```python
from build123d import *

# Parameters (mm, degrees)
SKETCH1_R               = 17.5
BOSS_EXTRUDE1_DEPTH     = 30
SKETCH5_R               = 10.95
CUT_EXTRUDE2_DEPTH      = 39.890873
SWEEP2_PITCH            = 10
SKETCH8_R               = 17.5
CUT_EXTRUDE3_DEPTH      = 41.699
SKETCH9_R               = 17.5
CUT_EXTRUDE4_DEPTH      = 39.890874
SKETCH10_W              = 40
SKETCH10_H              = 19.977262
BOSS_EXTRUDE2_DEPTH     = 40
SKETCH11_W              = 40
SKETCH11_H              = 19.977262
BOSS_EXTRUDE3_DEPTH     = 10
BOSS_EXTRUDE4_DEPTH     = 30
SKETCH14_R              = 1.905
CUT_EXTRUDE5_DEPTH      = 71.869594
SKETCH15_R              = 3.9243
CUT_EXTRUDE7_DEPTH      = 59.798031
SKETCH16_W              = 50
SKETCH16_H              = 19.977262
BOSS_EXTRUDE5_DEPTH     = 22
CUT_EXTRUDE8_DEPTH      = 12
BOSS_EXTRUDE6_DEPTH     = 19.977262
BOSS_EXTRUDE7_DEPTH     = 22
FILLET1_R               = 2
SKETCH21_W              = 7
SKETCH21_H              = 16
BOSS_EXTRUDE8_DEPTH     = 2
CUT_EXTRUDE9_DEPTH      = 76.769387
CUT_EXTRUDE9_DEPTH_BACK = 76.769387
SKETCH22_W              = 37.5
SKETCH22_H              = 30
SKETCH24_W              = 37.5
SKETCH24_H              = 30
BOSS_EXTRUDE9_DEPTH     = 12


with BuildPart() as part:
    # Sketch1 → Boss-Extrude1 (new body)
    with BuildSketch(Plane.XY):
        Circle(SKETCH1_R)
    extrude(amount=BOSS_EXTRUDE1_DEPTH)

    # Sketch5 → Cut-Extrude2 (cut, through all)
    with BuildSketch(Plane(origin=(0, 0, 0), x_dir=(-1, 0, 0), z_dir=(0, 0, -1))):
        Circle(SKETCH5_R)
    extrude(amount=-CUT_EXTRUDE2_DEPTH, mode=Mode.SUBTRACT)

    # Sweep2: arcs per turn and ends read off the stored shape
    # Sweep2: the profile of Sketch7 profile screwed along a right-hand helix through 3.75 turns, 16 arcs to a turn; built about Z, then put on its axis
    sweep2_z = Axis((0, 0, 0), (0, 0, 1))
    sweep2_corners = [(0, 7.7, 2.933013), (0, 10.9503, 4.809574), (0, 10.9503, 0.190426), (0, 7.7, 2.066987), (0, 7.45, 2.5)]
    with BuildLine(mode=Mode.PRIVATE) as sweep2_profile:
        Line(sweep2_corners[0], sweep2_corners[1])
        Line(sweep2_corners[1], sweep2_corners[2])
        Line(sweep2_corners[2], sweep2_corners[3])
        ThreePointArc((0, 7.7, 2.066987), (0, 7.516988, 2.25), (0, 7.45, 2.5))
        ThreePointArc((0, 7.45, 2.5), (0, 7.516988, 2.75), (0, 7.7, 2.933013))
    sweep2_cap = Face(sweep2_profile.wire())
    sweep2_arcs = [((0, 7.7, 2.066987), (0, 7.45, 2.211325), (0, 7.45, 2.5), (1, 0.8660254037844395, 1)), ((0, 7.45, 2.5), (0, 7.45, 2.788675), (0, 7.7, 2.933013), (1, 0.8660254037844395, 1))]  # start, shoulder, end, weights
    sweep2_turn_angles = [0, 11.25, 22.5, 33.75, 45, 56.25, 67.5, 78.75, 90, 101.25, 112.5, 123.75, 135, 146.25, 157.5, 168.75, 180, 191.25, 202.5, 213.75, 225, 236.25, 247.5, 258.75, 270, 281.25, 292.5, 303.75, 315, 326.25, 337.5, 348.75, 360]
    sweep2_turn_weights = [1, 0.9807852804032304, 1, 0.9807852804032304, 1, 0.9807852804032304, 1, 0.9807852804032304, 1, 0.9807852804032304, 1, 0.9807852804032304, 1, 0.9807852804032304, 1, 0.9807852804032304, 1, 0.9807852804032304, 1, 0.9807852804032304, 1, 0.9807852804032304, 1, 0.9807852804032304, 1, 0.9807852804032304, 1, 0.9807852804032304, 1, 0.9807852804032304, 1, 0.9807852804032304, 1]
    sweep2_turn_rails = [Edge.make_bspline([Vector(p[0], p[1], 0).rotate(sweep2_z, sweep2_turn_angles[k]) / sweep2_turn_weights[k] + Vector(0, 0, p[2] + SWEEP2_PITCH * sweep2_turn_angles[k] / 360) for k in range(33)], [0, 0, 0, 1, 1, 2, 2, 3, 3, 4, 4, 5, 5, 6, 6, 7, 7, 8, 8, 9, 9, 10, 10, 11, 11, 12, 12, 13, 13, 14, 14, 15, 15, 16, 16, 16], 2, sweep2_turn_weights) for p in sweep2_corners]
    sweep2_turn_sides = [*[Face.make_surface_from_curves(sweep2_turn_rails[p[0]], sweep2_turn_rails[p[1]]) for p in [(0, 1), (1, 2), (2, 3)]], *[Face.make_bezier_surface([[Vector(p[j][0], p[j][1], 0).rotate(sweep2_z, sweep2_turn_angles[2 * i + k]) / sweep2_turn_weights[2 * i + k] + Vector(0, 0, p[j][2] + SWEEP2_PITCH * sweep2_turn_angles[2 * i + k] / 360) for k in range(3)] for j in range(3)], [[p[3][j] * sweep2_turn_weights[2 * i + k] for k in range(3)] for j in range(3)]) for p in sweep2_arcs for i in range(16)]]
    sweep2_last_angles = [1080, 1091.25, 1102.5, 1113.75, 1125, 1136.25, 1147.5, 1158.75, 1170, 1181.25, 1192.5, 1203.75, 1215, 1226.25, 1237.5, 1248.75, 1260, 1271.25, 1282.5, 1293.75, 1305, 1316.25, 1327.5, 1338.75, 1350]
    sweep2_last_weights = [1, 0.9807852804032304, 1, 0.9807852804032304, 1, 0.9807852804032304, 1, 0.9807852804032304, 1, 0.9807852804032304, 1, 0.9807852804032304, 1, 0.9807852804032304, 1, 0.9807852804032304, 1, 0.9807852804032304, 1, 0.9807852804032304, 1, 0.9807852804032304, 1, 0.9807852804032304, 1]
    sweep2_last_rails = [Edge.make_bspline([Vector(p[0], p[1], 0).rotate(sweep2_z, sweep2_last_angles[k]) / sweep2_last_weights[k] + Vector(0, 0, p[2] + SWEEP2_PITCH * sweep2_last_angles[k] / 360) for k in range(25)], [0, 0, 0, 1, 1, 2, 2, 3, 3, 4, 4, 5, 5, 6, 6, 7, 7, 8, 8, 9, 9, 10, 10, 11, 11, 12, 12, 12], 2, sweep2_last_weights) for p in sweep2_corners]
    sweep2_last_sides = [*[Face.make_surface_from_curves(sweep2_last_rails[p[0]], sweep2_last_rails[p[1]]) for p in [(0, 1), (1, 2), (2, 3)]], *[Face.make_bezier_surface([[Vector(p[j][0], p[j][1], 0).rotate(sweep2_z, sweep2_last_angles[2 * i + k]) / sweep2_last_weights[2 * i + k] + Vector(0, 0, p[j][2] + SWEEP2_PITCH * sweep2_last_angles[2 * i + k] / 360) for k in range(3)] for j in range(3)], [[p[3][j] * sweep2_last_weights[2 * i + k] for k in range(3)] for j in range(3)]) for p in sweep2_arcs for i in range(12)]]
    sweep2 = Plane(origin=(0, 0, -10), x_dir=(-1, 0, 0), z_dir=(0, 0, 1)) * Solid(Shell([*[p.moved(Location((0, 0, SWEEP2_PITCH * i))) for i in range(3) for p in sweep2_turn_sides], *sweep2_last_sides, sweep2_cap, sweep2_cap.rotate(sweep2_z, 1350).moved(Location((0, 0, SWEEP2_PITCH * 1350 / 360)))]))
    add(sweep2)

    # Sketch8 → Cut-Extrude3 (cut, through all)
    with BuildSketch(Plane(origin=(0, 0, 0), x_dir=(-1, 0, 0), z_dir=(0, 0, -1))):
        with Locations(Location((0, 0, 0), (0, 0, 180))):
            Circle(SKETCH8_R)
    extrude(amount=CUT_EXTRUDE3_DEPTH, mode=Mode.SUBTRACT)

    # Sketch9 → Cut-Extrude4 (cut, through all)
    with BuildSketch(Plane.XY.offset(30)):
        Circle(SKETCH9_R)
    extrude(amount=CUT_EXTRUDE4_DEPTH, mode=Mode.SUBTRACT)



with BuildPart() as body_2:
    # Sketch10 → Boss-Extrude2 (new body)
    with BuildSketch(Plane(origin=(0, 0, 0), x_dir=(-1, 0, 0), z_dir=(0, 0, -1))):
        with Locations((0, -27.488631)):
            Rectangle(SKETCH10_W, SKETCH10_H)
    extrude(amount=-BOSS_EXTRUDE2_DEPTH)

    # Sketch11 → Boss-Extrude3 (add)
    with BuildSketch(Plane(origin=(0, 0, 0), x_dir=(-1, 0, 0), z_dir=(0, 0, -1))):
        with Locations((0, -27.488631)):
            Rectangle(SKETCH11_W, SKETCH11_H)
    extrude(amount=BOSS_EXTRUDE3_DEPTH)


with BuildPart() as part_1:
    add(part.part)

    add(body_2.part)  # Boss-Extrude4 merges body 2
    # Sketch13 → Boss-Extrude4 (add)
    with BuildSketch(Plane(origin=(0, 0, 0), x_dir=(-1, 0, 0), z_dir=(0, 0, -1))):
        with BuildLine():
            Line((0, -17.5), (-20, -17.5))
            Line((-20, -17.5), (-15.153881, -8.752707))
            ThreePointArc((-15.153881, -8.752707), (-8.748646, -15.156226), (0, -17.5))
        make_face()
    boss_extrude4 = extrude(amount=-BOSS_EXTRUDE4_DEPTH)

    # Mirror1: Boss-Extrude4 across plane
    add(boss_extrude4.mirror(Plane(origin=(0, 0, 0), x_dir=(0, 0, 1), z_dir=(1, 0, 0))))

    # Sketch14 → Cut-Extrude5 (cut, through all)
    with BuildSketch(Plane.XZ.offset(37.477262)):
        with Locations(Location((-10, 34.242642, 0), (0, 0, 270))):
            Circle(SKETCH14_R)
        with Locations(Location((10, 34.242642, 0), (0, 0, 270))):
            Circle(SKETCH14_R)
        with Locations(Location((-10, -4.242642, 0), (0, 0, 270))):
            Circle(SKETCH14_R)
        with Locations(Location((10, -4.242642, 0), (0, 0, 270))):
            Circle(SKETCH14_R)
    extrude(amount=-CUT_EXTRUDE5_DEPTH, mode=Mode.SUBTRACT)

    # Sketch15 → Cut-Extrude7 (cut, through all)
    with BuildSketch(Plane(origin=(0, -20.6734, 0), x_dir=(1, 0, 0), z_dir=(0, 1, 0))):
        with Locations(Location((-10, 4.242642, 0), (0, 0, 270))):
            Circle(SKETCH15_R)
        with Locations(Location((10, 4.242642, 0), (0, 0, 270))):
            Circle(SKETCH15_R)
        with Locations(Location((10, -34.242642, 0), (0, 0, 270))):
            Circle(SKETCH15_R)
        with Locations(Location((-10, -34.242642, 0), (0, 0, 270))):
            Circle(SKETCH15_R)
    extrude(amount=CUT_EXTRUDE7_DEPTH, mode=Mode.SUBTRACT)

    # Sketch16 → Boss-Extrude5 (add)
    with BuildSketch(Plane.ZY.offset(20)):
        with Locations((15, -27.488631)):
            Rectangle(SKETCH16_W, SKETCH16_H)
    extrude(amount=BOSS_EXTRUDE5_DEPTH)

    # Sketch17 → Cut-Extrude8 (cut)
    with BuildSketch(Plane.ZY.offset(37)):
        Polygon((4, -24.5), (8.5, -24.5), (8.5, -29.488888), (11, -29.488888), (11, -24.5), (26, -24.5), (26, -17.5), (4, -17.5), align=None)
    extrude(amount=-CUT_EXTRUDE8_DEPTH, mode=Mode.SUBTRACT)

    # Sketch19 → Boss-Extrude6 (add, through all)
    with BuildSketch(Plane(origin=(0, -17.5, 0), x_dir=(1, 0, 0), z_dir=(0, 1, 0))):
        Polygon((-42, -12), (-49, -12), (-49, -7), (-54, -7), (-54, -23), (-49, -23), (-49, -18), (-42, -18), align=None)
    extrude(amount=-BOSS_EXTRUDE6_DEPTH)

    # Sketch20 → Boss-Extrude7 (add)
    with BuildSketch(Plane(origin=(0, -17.5, 0), x_dir=(1, 0, 0), z_dir=(0, 1, 0))):
        Polygon((-54, -7), (-49, -7), (-49, -12), (-42, -12), (-42, -7), (-38.018198, -7), (-38.018198, -23), (-42, -23), (-42, -18), (-49, -18), (-49, -23), (-54, -23), align=None)
    extrude(amount=BOSS_EXTRUDE7_DEPTH)

    # Fillet1
    fillet1_edges = [part_1.edges().sort_by_distance(p)[0] for p in [
        (-42, -16.488631, 12),
        (-42, -16.488631, 18),
        (-49, -16.488631, 18),
        (-49, -16.488631, 12),
    ]]
    fillet(fillet1_edges, radius=FILLET1_R)

    # Sketch21 → Boss-Extrude8 (add)
    with BuildSketch(Plane.XZ.offset(37.477262)):
        with Locations((-45.5, 15)):
            Rectangle(SKETCH21_W, SKETCH21_H)
    extrude(amount=-BOSS_EXTRUDE8_DEPTH)

    # Sketch22 → Cut-Extrude9 (cut, two sides: drawn at the far end of the back side and taken through both)
    with BuildSketch(Plane(origin=(0, -17.5, 0), x_dir=(1, 0, 0), z_dir=(0, 1, 0)).offset(-CUT_EXTRUDE9_DEPTH_BACK)):
        with Locations((-1.25, -15)):
            Rectangle(SKETCH22_W, SKETCH22_H)
    extrude(amount=CUT_EXTRUDE9_DEPTH + CUT_EXTRUDE9_DEPTH_BACK, mode=Mode.SUBTRACT)

    # Sketch24 → Boss-Extrude9 (add)
    with BuildSketch(Plane.XZ.offset(37.477262)):
        with Locations((-1.25, 15)):
            Rectangle(SKETCH24_W, SKETCH24_H)
    extrude(amount=-BOSS_EXTRUDE9_DEPTH)


solid = part_1.part
```
Input: part model. Units: mm. Frame: model coordinates. A direction names the side the tool comes from. Coordinates: 2 decimals unless noted, no trailing zeros. Loops run counter-clockwise (first coordinate to the right, second up) from the corner with the lowest first, then second, coordinate; pieces in that order, holes last. Notation, with made-up numbers: M 21.5,-34.5 L 47.5,-34.5 A12 ccw 47.5,-22.5 Z; hole C -18,-2 d4. An arc over 180 degrees is marked long. Use a Markdown table: item, result. Add a question column.
1) Section D-D, the plane y = -1. Return the cut outline in (x, z).
2) Draft query along Z for faces 4 (the flat face through (-31, -21, 4)), 5 (the flat face through (-42, -26, 0)), 6 (the flat face through (18, -16, 0)). Return one class per face: +Z half, -Z half, draft (parallel to the pull), parting line (faces both ways), or undercut.
3) Set-up query: faces 1 (the flat face through (-45, -16, 18)), 2 (the flat face through (-12, -20.673, -5)), 3 (the flat face through (-46, -35.477, 10)). Return all of +Z, -Z, +X, -X, +Y, -Y with unobstructed straight access to the full face (end or side cutting, diameter ignored); none if empty.
4) Line query: L1, parallel to X at y = -20, z = 17; L2, parallel to X at y = -21.5, z = 25; L3, parallel to Z at x = 10, y = -18. Output: solid intervals per line, ascending. Write a range as from..to.
5) Pin query (flat end, axial travel): P1, Ø17.5, axis at y = -2, z = 15.5, coming from the +X side; P2, Ø6, axis at x = -29.5, z = 18, coming from the +Y side; P3, Ø2.5, axis at x = -46, y = -20.5, coming from the -Z side. Return the tip coordinate at first contact, or that it passes through.
6) Section A-A, the plane x = -10. Return the cut outline in (y, z), plus the area to 3 significant figures.
7) Section B-B, the plane z = 15.5. Return the cut outline in (x, y).
8) Section C-C, the plane y = -23.5. Return the cut outline in (x, z) (3 decimals).
Answer below:
| question | item | result |
|---|---|---|
| 1 | outline | M -54,7 L -49,7 L -49,10 A2 cw -47,12 L -44,12 A2 cw -42,10 L -42,7 L -38.02,7 L -38.02,23 L -42,23 L -42,20 A2 cw -44,18 L -47,18 A2 cw -49,20 L -49,23 L -54,23 Z |
| 2 | face 4 | undercut |
| 2 | face 5 | draft |
| 2 | face 6 | -Z half |
| 3 | face 1 | +Z, +Y |
| 3 | face 2 | +Y |
| 3 | face 3 | -Z, +Y |
| 4 | L1 | -54..-37, -25..-20, 17.5..20 |
| 4 | L2 | -42..-37, -25..-20, 17.5..20 |
| 4 | L3 | -10..-8.17, -0.32..0, 30..30.32, 38.17..40 |
| 5 | P1 | x = -38.02 |
| 5 | P2 | y = -24.5 |
| 5 | P3 | z = 11.98 |
| 6 | outline | M -37.48,-10 L -17.5,-10 L -17.5,-8.17 L -20.67,-8.17 L -20.67,-6.15 L -37.48,-6.15 Z; M -37.48,-2.34 L -20.67,-2.34 L -20.67,-0.32 L -17.5,-0.32 L -17.5,0 L -25.48,0 L -25.48,30 L -17.5,30 L -17.5,30.32 L -20.67,30.32 L -20.67,32.34 L -37.48,32.34 Z; M -37.48,36.15 L -20.67,36.15 L -20.67,38.17 L -17.5,38.17 L -17.5,40 L -37.48,40 Z |
| 6 | area | 582 mm2 |
| 7 | outline | M -54,-37.48 L 20,-37.48 L 20,-17.5 L 17.5,-12.99 L 17.5,-25.48 L -20,-25.48 L -20,-17.5 L -25,-17.5 L -25,-24.5 L -37,-24.5 L -37,-17.5 L -38.02,-17.5 L -38.02,4.5 L -54,4.5 Z |
| 8 | outline | M -54,7 L -49,7 L -49,10 A2 cw -47,12 L -44,12 A2 cw -42,10 L -42,-10 L 20,-10 L 20,40 L -42,40 L -42,20 A2 cw -44,18 L -47,18 A2 cw -49,20 L -49,23 L -54,23 Z; hole M -37,4 L -25,4 L -25,26 L -37,26 Z; hole M -20,0 L 17.5,0 L 17.5,30 L -20,30 Z; hole C -10,-4.243 d3.81; hole C -10,34.243 d3.81; hole C 10,-4.243 d3.81; hole C 10,34.243 d3.81 |
